from build123d import *

# Parameters (mm, degrees)
F0_W      = 133.858
F0_H      = 68.834
F1_DEPTH  = 17.78
F2_R      = 5.08
F3_W      = 123.698
F3_H      = 58.674
F4_DEPTH  = 7.62
F5_R      = 5.08
F6_R      = 3.040543
F6_W      = 2.994919
F6_H      = 8.357951
F6_W_2    = 5.08
F6_H_2    = 12.543548
F6_H_3    = 9.953398
F7_DEPTH  = 25.4
F8_W      = 35.758026
F8_H      = 4.692151
F9_DEPTH  = 25.4
F10_W     = 4.773868
F10_H     = 13.748736
F11_DEPTH = 25.4
F12_W     = 10.564138
F12_H     = 16.715713
F13_DEPTH = 25.4
F14_R     = 5.08


with BuildPart() as f1:
    # F0 (on Front) → F1 (new body)
    with BuildSketch(Plane.XZ):
        with Locations((2.471195, 34.417)):
            Rectangle(F0_W, F0_H)
    extrude(amount=F1_DEPTH)

    # F2
    f2_edges = [f1.edges().sort_by_distance(p)[0] for p in [
        (-64.457805, -8.89, 68.834),
        (69.400195, -8.89, 68.834),
        (69.400195, -8.89, 0),
        (-64.457805, -8.89, 0),
    ]]
    fillet(f2_edges, radius=F2_R)

    # F3 (on face) → F4 (cut)
    with BuildSketch(Plane.XZ.offset(17.78)):
        with Locations((2.471195, 34.417)):
            Rectangle(F3_W, F3_H)
    extrude(amount=-F4_DEPTH, mode=Mode.SUBTRACT)

    # F5
    f5_edges = [f1.edges().sort_by_distance(p)[0] for p in [
        (-59.377805, -13.97, 63.754),
        (-59.377805, -13.97, 5.08),
        (64.320195, -13.97, 63.754),
        (64.320195, -13.97, 5.08),
    ]]
    fillet(f5_edges, radius=F5_R)

    # F6 (on face) → F7 (cut)
    with BuildSketch(Plane.YZ.offset(69.400195)):
        with Locations((-13.613829, 10.810261)):
            Circle(F6_R)
        with Locations((-14.022106, 19.101335)):
            Rectangle(F6_W, F6_H)
        with Locations((-12.979566, 34.218168)):
            Rectangle(F6_W_2, F6_H_2)
        with Locations((-14.022106, 51.461173)):
            Rectangle(F6_W, F6_H_3)
    extrude(amount=-F7_DEPTH, mode=Mode.SUBTRACT)

    # F8 (on face) → F9 (cut)
    with BuildSketch(Plane(origin=(0, 0, 0), x_dir=(1, 0, 0), z_dir=(0, 0, -1))):
        with Locations((-34.609821, 13.577307)):
            Rectangle(F8_W, F8_H)
    extrude(amount=-F9_DEPTH, mode=Mode.SUBTRACT)

    # F10 (on face) → F11 (cut)
    with BuildSketch(Plane(origin=(-64.457805, 0, 0), x_dir=(0, -1, 0), z_dir=(-1, 0, 0))):
        with Locations((13.653257, 52.130621)):
            Rectangle(F10_W, F10_H)
    extrude(amount=-F11_DEPTH, mode=Mode.SUBTRACT)

    # F12 (on face) → F13 (cut)
    with BuildSketch(Plane(origin=(0, 0, 0), x_dir=(-1, 0, 0), z_dir=(0, 1, 0))):
        with Locations((49.606802, 53.344105)):
            Rectangle(F12_W, F12_H)
    extrude(amount=-F13_DEPTH, mode=Mode.SUBTRACT)

    # F14
    f14_edges = [f1.edges().sort_by_distance(p)[0] for p in [
        (-54.888871, -5.08, 61.701961),
        (-54.888871, -5.08, 44.986248),
        (-44.324733, -5.08, 44.986248),
        (-44.324733, -5.08, 61.701961),
    ]]
    fillet(f14_edges, radius=F14_R)


solid = f1.part
For this review, take the finished solid that the model builds, in its own axes (mm). A direction names the side the tool comes from. Round coordinates to 2 decimals unless told otherwise and drop trailing zeros. Order: outer loops, then holes, each group sorted by start corner. A loop starts at its lowest first (then second) coordinate and runs counter-clockwise, first axis right, second up. Notation, with made-up numbers: (4, -24.75) -> (51, -24.75) arc R32 cw to (51, 10.25) -> close; hole circle Ø7 at (-29, 37). An arc over 180 degrees is marked (long way). Write item = value, one per line. Start each with the question number.
1) To check wall thickness, follow line 1 (Z direction, x = -19.5, y = -10.75); line 2 (X direction, y = -13, z = 26.5); line 3 (Y direction, x = -44.5, z = 4.5). State the ranges of each line that lie inside material, in increasing order. Write a range as from..to.
2) Take a section at A-A on z = 22. State the section outline as (x, y) points, plus the area to 3 significant figures.
3) Take a section at D-D on x = -48. State the section outline as (y, z) points, plus the area to 3 significant figures.
4) Insertion check: pin 1 (10 mm diameter, centred on x = 34.5, z = 40.5, fed in from -Y); pin 2 (5 mm diameter, centred on y = -14.5, z = 1.5, fed in from -X). Each pin has a flat end and moves straight along its axis. Give the tip position at first contact, or say it passes through.
5) Tool access review of faces 4 (the face through (67, -14, 56.438)), 5 (the face through (-44.325, -5, 53)), 6 (the face through (67, -13, 27.946)), 7 (the face through (2, -14, 63.754)), 8 (the face through (-62, -16.04, 52)): name each direction out of +Z, -Z, +X, -X, +Y, -Y from which nothing blocks a thin tool from reaching the whole face with its end or side.
6) Take a section at C-C on x = -29.5. State the section outline as (y, z) points.
7) The part is to be moulded in two halves that separate along Z. For faces 1 (the face through (2, -9, 68.834)), 2 (the face through (-3, -17.78, 4)), 3 (the face through (67, -15.52, 19)), say which applies: +Z half, -Z half, draft (parallel to the pull), parting line (faces both ways), or undercut.
8) Take a section at B-B on y = -5.25. State the section outline as (x, z) points.
Verdict:
q1.line_1 = 0..5.08, 63.75..68.83
q1.line_2 = -64.46..-59.38, 64.32..69.4
q1.line_3 = -17.78..-15.92, -11.23..0
q2.outline = (-64.46, -17.78) -> (-59.38, -17.78) -> (-59.38, -10.16) -> (64.32, -10.16) -> (64.32, -12.52) -> (69.4, -12.52) -> (69.4, 0) -> (-64.46, 0) -> close; (64.32, -17.78) -> (69.4, -17.78) -> (69.4, -15.52) -> (64.32, -15.52) -> close
q2.area = 1,420 mm2
q3.outline = (-17.78, 0) -> (-15.92, 0) -> (-15.92, 5.08) -> (-17.78, 5.08) -> close; (-17.78, 63.75) -> (-10.16, 63.75) -> (-10.16, 61.5) -> (0, 61.5) -> (0, 68.83) -> (-17.78, 68.83) -> close; (-11.23, 0) -> (0, 0) -> (0, 45.18) -> (-10.16, 45.18) -> (-10.16, 5.08) -> (-11.23, 5.08) -> close
q3.area = 587 mm2
q4.pin_1 = -10.16
q4.pin_2 = -64.34
q5.face_4 = +X, -X
q5.face_5 = +Y, -Y
q5.face_6 = +X
q5.face_7 = -Y
q5.face_8 = -X
q6.outline = (-17.78, 0) -> (-15.92, 0) -> (-15.92, 5.08) -> (-17.78, 5.08) -> close; (-17.78, 63.75) -> (-10.16, 63.75) -> (-10.16, 5.08) -> (-11.23, 5.08) -> (-11.23, 0) -> (0, 0) -> (0, 68.83) -> (-17.78, 68.83) -> close
q7.face_1 = +Z half
q7.face_2 = draft
q7.face_3 = undercut
q8.outline = (-64.46, 5.08) arc R5.08 ccw to (-59.38, 0) -> (64.32, 0) arc R5.08 ccw to (69.4, 5.08) -> (69.4, 63.75) arc R5.08 ccw to (64.32, 68.83) -> (-59.38, 68.83) arc R5.08 ccw to (-64.46, 63.75) -> close; hole (-54.89, 50.07) arc R5.08 ccw to (-49.81, 44.99) -> (-49.4, 44.99) arc R5.08 ccw to (-44.32, 50.07) -> (-44.32, 56.62) arc R5.08 ccw to (-49.4, 61.7) -> (-49.81, 61.7) arc R5.08 ccw to (-54.89, 56.62) -> close
